Solid Edge part; units mm, degrees
sketch "Sketch1" plane through (0, 0, 0) normal (0, -1, 0) x (1, 0, 0)
  circle A0 centre (0, 0) radius 3.175
  line L0 (-2.5981, 4.5) -> (-5.1962, 0)
  line L1 (-5.1962, 0) -> (-2.5981, -4.5)
  line L2 (-2.5981, -4.5) -> (2.5981, -4.5)
  line L3 (2.5981, -4.5) -> (5.1962, 0)
  line L4 (5.1962, 0) -> (2.5981, 4.5)
  line L5 (2.5981, 4.5) -> (-2.5981, 4.5)
extrude "Protrusion1" add sketch "Sketch1" against normal blind 3.5
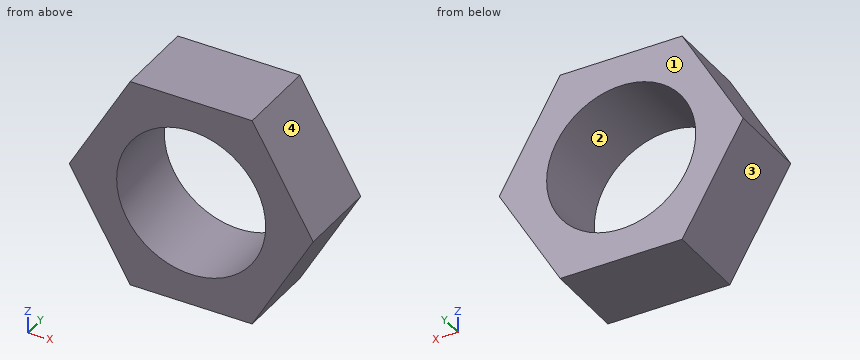
Geometry check sheet. Reference: the model listing, model coordinates, mm. Face numbers are marked on the shaded views. Coordinates: 2 decimals unless noted, no trailing zeros. Order: outer loops, then holes, each group sorted by start corner. A loop starts at its lowest first (then second) coordinate and runs counter-clockwise, first axis right, second up. Notation, with made-up numbers: (51, 60) - (110, 60) arc R38 ccw to (110, 99) - close; hole circle Ø9 at (-12, 81). An arc over 180 degrees is marked (long way). Answer in a Markdown table with one row per item. Add a question column.
1) Release check for a two-part mould opening along X. For the marked faces 1, 2, 3 and 4 record: +X half, -X half, draft (parallel to the pull), parting line (faces both ways), or undercut.
2) Material ranges on line 1 along Z through (x, y) = (0, 2.15) (3 decimals); line 2 along Z through (x, y) = (-2, 1.9); line 3 along X through (y, z) = (2.3, 1.25), recorded low to high. Write a range as [from, to].
3) Cross-section at B-B, the plane z = -2.5. Record the cut outline in (x, y), then the cut area to 3 significant figures.
4) Gauge pin test, flat end, axial feed: P1, Ø1.5, axis at x = -4, y = 2.5, coming from the -Z side. Record the tip position at first contact, or that the pin passes through.
5) Cross-section at A-A, the plane x = 0. Record the cut outline in (y, z) (3 decimals).
6) Cross-section at C-C, the plane y = 2.85. Record the cut outline in (x, z) (3 decimals).
Check result:
| question | item | result |
|---|---|---|
| 1 | face 1 | draft |
| 1 | face 2 | undercut |
| 1 | face 3 | -X half |
| 1 | face 4 | +X half |
| 2 | line 1 | z = [-4.5, -3.175], [3.175, 4.5] |
| 2 | line 2 | z = [-4.5, -2.47], [2.47, 4.5] |
| 2 | line 3 | x = [-4.47, -2.92], [2.92, 4.47] |
| 3 | outline | (-3.75, 0) - (-1.96, 0) - (-1.96, 3.5) - (-3.75, 3.5) - close; (1.96, 0) - (3.75, 0) - (3.75, 3.5) - (1.96, 3.5) - close |
| 3 | area | 12.6 mm² |
| 4 | P1 | stops at z = -3.37 |
| 5 | outline | (0, -4.5) - (3.5, -4.5) - (3.5, -3.175) - (0, -3.175) - close; (0, 3.175) - (3.5, 3.175) - (3.5, 4.5) - (0, 4.5) - close |
| 6 | outline | (-5.196, 0) - (-2.598, -4.5) - (2.598, -4.5) - (5.196, 0) - (2.598, 4.5) - (-2.598, 4.5) - close; hole circle Ø6.35 at (0, 0) |
